Autodesk Inventor part; units mm, degrees
ref_plane "YZ Plane" through (0, 0, 0) normal (1, 0, 0) x (0, 1, 0)
ref_plane "XZ Plane" through (0, 0, 0) normal (0, 1, 0) x (-1, 0, 0)
ref_plane "XY Plane" through (0, 0, 0) normal (0, 0, 1) x (1, 0, 0)
sketch "Esquisse1" plane through (0, 0, 0) normal (0, 0, 1) x (1, 0, 0)
  line L0 (-24.5097, 12.7546) -> (-9.5097, 12.7546)
  line L1 (-9.5097, 12.7546) -> (-9.5097, -2.2454)
  line L2 (-9.5097, -2.2454) -> (-24.5097, -2.2454)
  line L3 (-24.5097, -2.2454) -> (-24.5097, 0.7546)
  line L4 (-24.5097, 0.7546) -> (-12.5097, 0.7546)
  line L5 (-12.5097, 0.7546) -> (-12.5097, 3.7546)
  line L6 (-12.5097, 3.7546) -> (-24.5097, 3.7546)
  line L7 (-24.5097, 3.7546) -> (-24.5097, 12.7546)
  dimension "d0" = 15
  dimension "d1" = 15
  dimension "d2" = 3
  dimension "d3" = 9
  dimension "d4" = 12
extrude "Extrusion1" add sketch "Esquisse1" along normal blind 20
sketch "Esquisse2" plane through (-24.5097, 12.7546, 0) normal (0, 1, 0) x (1, 0, 0)
  circle A0 centre (3, -3) radius 1.5
  circle A1 centre (3, -17) radius 1.5
  line L0 (0, 0) -> (0, -20)
  line L1 (15, 0) -> (0, 0)
  line L2 (15, -20) -> (0, -20)
  point P0 (24.5097, 0)
  dimension "d8" = 3
  dimension "d9" = 3
  dimension "d13" = 3
  dimension "d15" = 3
  dimension "d30" = 3
  dimension "d31" = 3
hole "Perçage1" at (-21.5097, 12.7546, 3) at (-21.5097, 12.7546, 17) direction (0, -1, 0) diameter 3 end through all
sketch "Esquisse3" plane through (-24.5097, 12.7546, 0) normal (0, 1, 0) x (1, 0, 0)
  circle A0 centre (7.5, -9.6122) radius 4
  line L0 (15, 0) -> (15, -20)
  point P0 (24.5097, 0)
  dimension "d26" = 8
  dimension "d27" = 7.5
extrude "Extrusion2" cut sketch "Esquisse3" against normal blind 7
fillet "Congé1" radius 1 6 edges at (-12.5097, 3.7546, 10) (-12.5097, 0.7546, 10) (-24.5097, -2.2454, 10) (-24.5097, 0.7546, 10) (-24.5097, 3.7546, 10) (-24.5097, 12.7546, 10)
properties part number "support tige voiture"
The listing builds one solid part. Answer for the finished solid, in the listing's coordinates (mm). A direction names the side the tool comes from. Give positions to 0.01 mm unless a question says otherwise; leave off trailing zeros. Order: outer loops, then holes, each group sorted by start corner. A loop starts at its lowest first (then second) coordinate and runs counter-clockwise, first axis right, second up. Notation, with made-up numbers: (-10, 22) -> (14, 22) arc R24 cw to (14, 42) -> close; hole circle Ø9 at (89, -27). An arc over 180 degrees is marked (long way). Put each result on its own line as item: value.
Item 1: A cutting plane is placed at A-A on z = 3. Give the vertices of the cut face in (x, y).
Established:
outline: (-24.51, -1.25) arc R1 ccw to (-23.51, -2.25) -> (-23.01, -2.25) -> (-23.01, 0.75) -> (-23.51, 0.75) arc R1 ccw to (-24.51, -0.25) -> close; (-24.51, 4.75) arc R1 ccw to (-23.51, 3.75) -> (-23.01, 3.75) -> (-23.01, 12.75) -> (-23.51, 12.75) arc R1 ccw to (-24.51, 11.75) -> close; (-20.01, -2.25) -> (-9.51, -2.25) -> (-9.51, 12.75) -> (-20.01, 12.75) -> (-20.01, 3.75) -> (-13.51, 3.75) arc R1 cw to (-12.51, 2.75) -> (-12.51, 1.75) arc R1 cw to (-13.51, 0.75) -> (-20.01, 0.75) -> close
Item 2: For a pull along X with two mould halves and no side action, classify faces 4 (the face through (-20.045, 8.192, 2.675)), 5 (the face through (-20.045, -0.766, 2.675)), 6 (the face through (-13, 12.755, 8)), 7 (the face through (-24.51, 8, 10)) as released by +X, released by -X, zero draft, split by the parting line, or undercut.
Established:
face 4: undercut
face 5: undercut
face 6: zero draft
face 7: released by -X
Item 3: A cutting plane is placed at C-C on z = 14.75. Give the vertices of the cut face in (x, y), plus the area to 3 significant figures.
Established:
outline: (-24.51, -1.25) arc R1 ccw to (-23.51, -2.25) -> (-9.51, -2.25) -> (-9.51, 12.75) -> (-23.51, 12.75) arc R1 ccw to (-24.51, 11.75) -> (-24.51, 4.75) arc R1 ccw to (-23.51, 3.75) -> (-13.51, 3.75) arc R1 cw to (-12.51, 2.75) -> (-12.51, 1.75) arc R1 cw to (-13.51, 0.75) -> (-23.51, 0.75) arc R1 ccw to (-24.51, -0.25) -> close
area: 189 mm^2
Item 4: Given P1, Ø0.5, axis at y = 2, z = 7.5, coming from the -X side; P2, Ø1.8, axis at x = -21.51, z = 17, coming from the -Y side; P3, Ø4, axis at x = -15.5, z = 9.5, coming from the +Y side, each flat-ended and moving along its own axis, determine where each tip first touches the part or whether it passes through.
Established:
P1: stops at x = -12.51
P2: passes through
P3: stops at y = 5.75
Item 5: A cutting plane is placed at D-D on x = -20.75. Give the vertices of the cut face in (y, z).
Established:
outline: (-2.25, 0) -> (0.75, 0) -> (0.75, 1.71) -> (-2.25, 1.71) -> close; (-2.25, 4.29) -> (0.75, 4.29) -> (0.75, 15.71) -> (-2.25, 15.71) -> close; (-2.25, 18.29) -> (0.75, 18.29) -> (0.75, 20) -> (-2.25, 20) -> close; (3.75, 0) -> (12.75, 0) -> (12.75, 1.71) -> (3.75, 1.71) -> close; (3.75, 4.29) -> (12.75, 4.29) -> (12.75, 8.19) -> (5.75, 8.19) -> (5.75, 11.03) -> (12.75, 11.03) -> (12.75, 15.71) -> (3.75, 15.71) -> close; (3.75, 18.29) -> (12.75, 18.29) -> (12.75, 20) -> (3.75, 20) -> close
Item 6: A cutting plane is placed at B-B on y = 6.25. Give the vertices of the cut face in (x, z).
Established:
outline: (-24.51, 0) -> (-9.51, 0) -> (-9.51, 20) -> (-24.51, 20) -> close; hole circle Ø3 at (-21.51, 3); hole circle Ø3 at (-21.51, 17); hole circle Ø8 at (-17.01, 9.61)
Item 7: For faces 1 (the face through (-12.81, 1.04, 10.14)), 2 (the face through (-13.194, 9.304, 8.411)), 3 (the face through (-24.21, 12.47, 10.14)), determine the directions among +Z, -Z, +X, -X, +Y, -Y from which every point of the face is accessible in a straight line to the end or side of a thin tool.
Established:
face 1: +Z, -Z, -X
face 2: +Y
face 3: +Z, -Z, -X, +Y
Item 8: Straight lines are drawn through the part: line 1 (Y direction, x = -15, z = 12.5); line 2 (X direction, y = 6.25, z = 3); line 3 (Z direction, x = -22.5, y = 0). For each, find the intervals that lie inside material, in ascending order.
Established:
line 1: y = -2.25 to 0.75, 3.75 to 5.75
line 2: x = -24.51 to -23.01, -20.01 to -9.51
line 3: z = 0 to 1.87, 4.13 to 15.87, 18.13 to 20
